Check sheet for the modelled part. Datum: model origin and axes. Units: mm. Coordinates: 2 decimals unless noted, no trailing zeros. Loops run counter-clockwise (first coordinate to the right, second up) from the corner with the lowest first, then second, coordinate; pieces in that order, holes last. Notation, with made-up numbers: M -35.75,-22 L 23.25,-22 A29 cw 23.25,-1 Z; hole C -3,33 d6. An arc over 180 degrees is marked long. Use CSV: the item, a comma, the result in double quotes. Start each with the question number.
(1) Draft check along X on faces 1 (the cylindrical face through (23.846, -9.86, 7.509)), 2 (the conical face through (1.06, -19.68, 48.31)), 3 (the flat face through (-1, 0, -125)). Enter one of: pulls with the +X half, pulls with the -X half, needs draft (parallel to the pull), parting line crosses it, or undercut.
(2) Section check B-B on x = 0. Record the cut outline in (y, z).
(3) Section check A-A on y = -14.5. Record the cut outline in (x, z).
(4) Section check C-C on x = 19. Give the number of separate pieces and of enclosed holes in the cut face, and give its area (3 significant figures).
(5) Scan lines: line 1 (Z direction, x = 0, y = -15); line 2 (Z direction, x = -2.5, y = -6.25); line 3 (X direction, y = -8.25, z = -11.5). Record each from-to range of solid material in increasing order.
(6) Go/stop test with flat-tipped pins: pin 1 Ø1.5 at (x, y) = (-33, -14) entering from +Z; pin 2 Ø2 at (x, y) = (-23, -5) entering from +Z; pin 3 Ø8 at (x, y) = (4, -16.5) entering from -Z. Record where each tip stops, or that it passes through.
from build123d import *

# Parameters (mm, degrees)
F0_R     = 25
F1_DEPTH = 20
F2_SIZE2 = 2
F2_SIZE  = 2


with BuildPart() as f1:
    # F0 (on Front) → F1 (new body)
    with BuildSketch(Plane.XZ):
        with BuildLine():
            ThreePointArc((50, 0), (0, 50), (-50, 0))
            Line((-50, 0), (-50, -255))
            ThreePointArc((-50, -255), (0, -305), (50, -255))
            Line((50, -255), (50, 0))
        make_face()
        with Locations((0, -255)):
            Circle(F0_R, mode=Mode.SUBTRACT)
        Circle(F0_R, mode=Mode.SUBTRACT)
    extrude(amount=F1_DEPTH)

    # F2
    f2_edges = [f1.edges().sort_by_distance(p)[0] for p in [
        (-50, -20, -127.5),
        (0, -20, 50),
        (50, -20, -127.5),
        (0, -20, -305),
        (0, 0, -305),
        (-50, 0, -127.5),
        (0, 0, 50),
        (50, 0, -127.5),
    ]]
    chamfer(f2_edges, length=F2_SIZE, length2=F2_SIZE2)


solid = f1.part
Outcome:
1,face 1,"undercut"
1,face 2,"parting line crosses it"
1,face 3,"needs draft"
2,outline,"M -20,-303 L -18,-305 L -2,-305 L 0,-303 L 0,-280 L -20,-280 Z; M -20,-230 L 0,-230 L 0,-25 L -20,-25 Z; M -20,25 L 0,25 L 0,48 L -2,50 L -18,50 L -20,48 Z"
3,outline,"M -50,-255 A50 ccw 50,-255 L 50,0 A50 ccw -50,0 Z; hole C 0,-255 d50; hole C 0,0 d50"
4,separate pieces,"3"
4,enclosed holes,"0"
4,area,"5,640 mm²"
5,line 1,"z = -305 to -280, -230 to -25, 25 to 50"
5,line 2,"z = -304.94 to -279.87, -230.13 to -24.87, 24.87 to 49.94"
5,line 3,"x = -50 to -22.2, 22.2 to 50"
6,pin 1,"stops at z = 38.21"
6,pin 2,"stops at z = 44.9"
6,pin 3,"stops at z = -305"
